```python
from build123d import *

# Parameters (mm, degrees)
BOX052_W          = 10
BOX052_H          = 12
BOX052_DEPTH      = 6
BOX053_W          = 10
BOX053_H          = 12
BOX053_DEPTH      = 6
CYLINDER011_R     = 1.49
CYLINDER011_DEPTH = 10
ARRAY017_Y_COUNT  = 5
ARRAY017_Y_PITCH  = 7.58
BOX051_W          = 10
BOX051_H          = 10
BOX051_DEPTH      = 31
BOX050_W          = 10
BOX050_H          = 10
BOX050_DEPTH      = 30
BOX049_W          = 10
BOX049_H          = 10
BOX049_DEPTH      = 25
BOX048_W          = 10
BOX048_H          = 10
BOX048_DEPTH      = 25
BOX046_W          = 2
BOX046_H          = 80
BOX046_DEPTH      = 18
BOX047_W          = 4
BOX047_H          = 76
BOX047_DEPTH      = 18


with BuildPart() as usb:
    # Box052 → Box052 (new body)
    with BuildSketch(Plane(origin=(110, 5, 4), x_dir=(1, 0, 0), z_dir=(0, 0, 1))):
        with Locations((5, 6)):
            Rectangle(BOX052_W, BOX052_H)
    extrude(amount=BOX052_DEPTH)


with BuildPart() as obj1:
    # Box053 → Box053 (new body)
    with BuildSketch(Plane(origin=(110, 19, 5.5), x_dir=(1, 0, 0), z_dir=(0, 0, 1))):
        with Locations((5, 6)):
            Rectangle(BOX053_W, BOX053_H)
    extrude(amount=BOX053_DEPTH)


with BuildPart() as fusion008032:
    # Cylinder011 → Cylinder011 (new body)
    with BuildSketch(Plane(origin=(143, 6, 13), x_dir=(0, 0, -1), z_dir=(1, 0, 0))):
        Circle(CYLINDER011_R)
    extrude(amount=CYLINDER011_DEPTH)

    # Array017 Y: Fusion008032 ×5


with BuildPart() as fusion008032_1:
    add(fusion008032.part)
    with Locations(*[(0, i * ARRAY017_Y_PITCH, 0) for i in range(1, ARRAY017_Y_COUNT)]):
        add(fusion008032.part)


with BuildPart() as fusion008032_2:
    # Array017 placement: moved
    add(fusion008032_1.part.moved(Location((-33, 39, 0))))

    # Fusion008032: union USB, obj1
    add(usb.part)
    add(obj1.part)


with BuildPart() as obj2:
    # Box051 → Box051 (new body)
    with BuildSketch(Plane(origin=(110, 80.8, 0), x_dir=(1, 0, 0), z_dir=(0, 0, 1))):
        with Locations((5, 5)):
            Rectangle(BOX051_W, BOX051_H)
    extrude(amount=BOX051_DEPTH)


with BuildPart() as obj3:
    # Box050 → Box050 (new body)
    with BuildSketch(Plane(origin=(109, -8.8, 0), x_dir=(1, 0, 0), z_dir=(0, 0, 1))):
        with Locations((5, 5)):
            Rectangle(BOX050_W, BOX050_H)
    extrude(amount=BOX050_DEPTH)


with BuildPart() as obj4:
    # Box049 → Box049 (new body)
    with BuildSketch(Plane(origin=(114.8, 78.8, 0), x_dir=(1, 0, 0), z_dir=(0, 0, 1))):
        with Locations((5, 5)):
            Rectangle(BOX049_W, BOX049_H)
    extrude(amount=BOX049_DEPTH)


with BuildPart() as obj5:
    # Box048 → Box048 (new body)
    with BuildSketch(Plane(origin=(114.8, -6.8, 0), x_dir=(1, 0, 0), z_dir=(0, 0, 1))):
        with Locations((5, 5)):
            Rectangle(BOX048_W, BOX048_H)
    extrude(amount=BOX048_DEPTH)


with BuildPart() as obj6:
    # Box046 → Box046 (new body)
    with BuildSketch(Plane(origin=(113, 1, 23), x_dir=(1, 0, 0), z_dir=(0, 0, 1))):
        with Locations((1, 40)):
            Rectangle(BOX046_W, BOX046_H)
    extrude(amount=BOX046_DEPTH)


with BuildPart() as front_cpu:
    # Box047 → Box047 (new body)
    with BuildSketch(Plane(origin=(113, 3, 23), x_dir=(1, 0, 0), z_dir=(0, 0, 1))):
        with Locations((2, 38)):
            Rectangle(BOX047_W, BOX047_H)
    extrude(amount=BOX047_DEPTH)

    # Fusion008031: union obj6
    add(obj6.part)


with BuildPart() as front_cpu_1:
    # Fusion008031 placement: moved
    add(front_cpu.part.moved(Location((0, 0, -19))))

    # Cut047: cut obj5
    add(obj5.part, mode=Mode.SUBTRACT)

    # Cut048: cut obj4
    add(obj4.part, mode=Mode.SUBTRACT)

    # Cut049: cut obj3
    add(obj3.part, mode=Mode.SUBTRACT)

    # Cut050: cut obj2
    add(obj2.part, mode=Mode.SUBTRACT)

    # Cut053: cut Fusion008032
    add(fusion008032_2.part, mode=Mode.SUBTRACT)


solid = front_cpu_1.part
```
The listing builds one solid part. Answer for the finished solid, in the listing's coordinates (mm). A direction names the side the tool comes from. Give positions to 0.01 mm unless a question says otherwise; leave off trailing zeros. Loops run counter-clockwise (first coordinate to the right, second up) from the corner with the lowest first, then second, coordinate; pieces in that order, holes last. Notation, with made-up numbers: (85.5, 2.25) - (109.5, 2.25) arc R16 ccw to (109.5, 26.25) - close; hole circle Ø11 at (34.25, 47). An arc over 180 degrees is marked (long way). Return JSON: item names as keys, results as strings. Group by question number.
1. Determine the mould class of faces 6 (the flat face through (115, 42, 22)), 7 (the flat face through (115, 17, 7)), 8 (the cylindrical face through (114.97, 59.25, 14.18)), 9 (the flat face through (115, 11, 10)) for opening direction Z: pulls with the +Z half, pulls with the -Z half, needs draft (parallel to the pull), parting line crosses it, or undercut.
2. Find section A-A (y = 22). Write down the section's boundary in (x, z), then the cut area to 3 significant figures.
3. Straight lines are drawn through the part: line 1 (Y direction, x = 114.45, z = 13); line 2 (Y direction, x = 115.15, z = 9.25); line 3 (Y direction, x = 115.6, z = 13). For each, find the intervals that lie inside material, in ascending order. Write a range as [from, to].
4. Find section C-C (x = 114). Write down the section's boundary in (y, z).
5. Find section B-B (z = 8.5). Write down the section's boundary in (x, y).
6. Which of the six approach directions +Z, -Z, +X, -X, +Y, -Y give full straight-line access (tool end or side, diameter ignored) to faces 1 (the flat face through (115, 49, 4)), 2 (the flat face through (115, 19, 8)), 3 (the flat face through (113, 40, 13)), 4 (the flat face through (114.8, 80, 13)), 5 (the flat face through (114.8, 2, 13))?
7. Given pin 1 Ø1 at (y, z) = (80, 15) entering from +X; pin 2 Ø2 at (x, z) = (116, 19) entering from +Y; pin 3 Ø2 at (x, y) = (115.5, 10) entering from -Z, each flat-ended and moving along its own axis, determine where each tip first touches the part or whether it passes through.
8. Find section D-D (z = 13). Write down the section's boundary in (x, y).
Verdict:
{
 "1": {"face 6": "pulls with the +Z half", "face 7": "needs draft", "face 8": "undercut", "face 9": "pulls with the -Z half"},
 "2": {"outline": "(113, 4) - (117, 4) - (117, 5.5) - (113, 5.5) - close; (113, 11.5) - (117, 11.5) - (117, 22) - (113, 22) - close", "area": "48.0 mm^2"},
 "3": {"line 1": "y = [1.2, 43.51], [46.49, 51.09], [54.07, 58.67], [61.65, 66.25], [69.23, 73.83], [76.81, 80.8]", "line 2": "y = [3.2, 5], [17, 19], [31, 78.8]", "line 3": "y = [3.2, 43.51], [46.49, 51.09], [54.07, 58.67], [61.65, 66.25], [69.23, 73.83], [76.81, 78.8]"},
 "4": {"outline": "(1.2, 4) - (5, 4) - (5, 10) - (17, 10) - (17, 4) - (80.8, 4) - (80.8, 22) - (1.2, 22) - close; hole (19, 5.5) - (31, 5.5) - (31, 11.5) - (19, 11.5) - close; hole circle Ø2.98 at (45, 13); hole circle Ø2.98 at (52.58, 13); hole circle Ø2.98 at (60.16, 13); hole circle Ø2.98 at (67.74, 13); hole circle Ø2.98 at (75.32, 13)"},
 "5": {"outline": "(113, 1.2) - (114.8, 1.2) - (114.8, 3.2) - (117, 3.2) - (117, 5) - (113, 5) - close; (113, 17) - (117, 17) - (117, 19) - (113, 19) - close; (113, 31) - (117, 31) - (117, 78.8) - (114.8, 78.8) - (114.8, 80.8) - (113, 80.8) - close"},
 "6": {"face 1": "-Z, +X, -X, +Y, -Y", "face 2": "+X, -X", "face 3": "+Z, -Z, -X, +Y, -Y", "face 4": "+Z, -Z, +X, +Y", "face 5": "+Z, -Z, +X, -Y"},
 "7": {"pin 1": "stops at x = 114.8", "pin 2": "stops at y = 78.8", "pin 3": "stops at z = 10"},
 "8": {"outline": "(113, 1.2) - (114.8, 1.2) - (114.8, 3.2) - (117, 3.2) - (117, 43.51) - (113, 43.51) - close; (113, 46.49) - (117, 46.49) - (117, 51.09) - (113, 51.09) - close; (113, 54.07) - (117, 54.07) - (117, 58.67) - (113, 58.67) - close; (113, 61.65) - (117, 61.65) - (117, 66.25) - (113, 66.25) - close; (113, 69.23) - (117, 69.23) - (117, 73.83) - (113, 73.83) - close; (113, 76.81) - (117, 76.81) - (117, 78.8) - (114.8, 78.8) - (114.8, 80.8) - (113, 80.8) - close"}
}
